For this review, use the dimensioned drawing (mm, ordinates from the lowest corner) and the shaded views. Give positions to 0.01 mm unless a question says otherwise; leave off trailing zeros. Loops run counter-clockwise (first coordinate to the right, second up) from the corner with the lowest first, then second, coordinate; pieces in that order, holes last. Notation, with made-up numbers: (66.25, -23.75) -> (90.25, -23.75) arc R19 ccw to (90.25, -5.75) -> close; hole circle Ø1 at (82, -29.5). An arc over 180 degrees is marked (long way). Use a Markdown table: item, result. Add a question column.
1. Add section B-B (y = 6.3). State the section outline as (x, z) points, and give its area (3 significant figures).
2. For pin 1 Ø4 at (y, z) = (8.5, 6.5) entering from -X; pin 2 Ø1.5 at (x, z) = (6, 2.5) entering from -Y; pin 3 Ø1.8 at (y, z) = (6.3, 7) entering from +X; pin 4 Ø1 at (y, z) = (6, 6) entering from -X, all flat-tipped, find the tip position at first contact; note any pin that passes through.
3. Add section D-D (y = 9). State the section outline as (x, z) points, and give its area (3 significant figures).
4. To check wall thickness, follow line 1 (Y direction, x = 6.75, z = 7); line 2 (Z direction, x = 3.75, y = 6.3); line 3 (X direction, y = 2, z = 5.5). State the ranges of each line that lie inside material, in increasing order.
5. Add section C-C (x = 6.75). State the section outline as (y, z) points.
6. Add section A-A (z = 7). State the section outline as (x, y) points, and give its area (3 significant figures).
7. Draft analysis for pull direction Y (two halves, no side actions). For the marked faces 1, 2 and 3, state which applies: pulls with the +Y half, pulls with the -Y half, needs draft (parallel to the pull), parting line crosses it, or undercut.
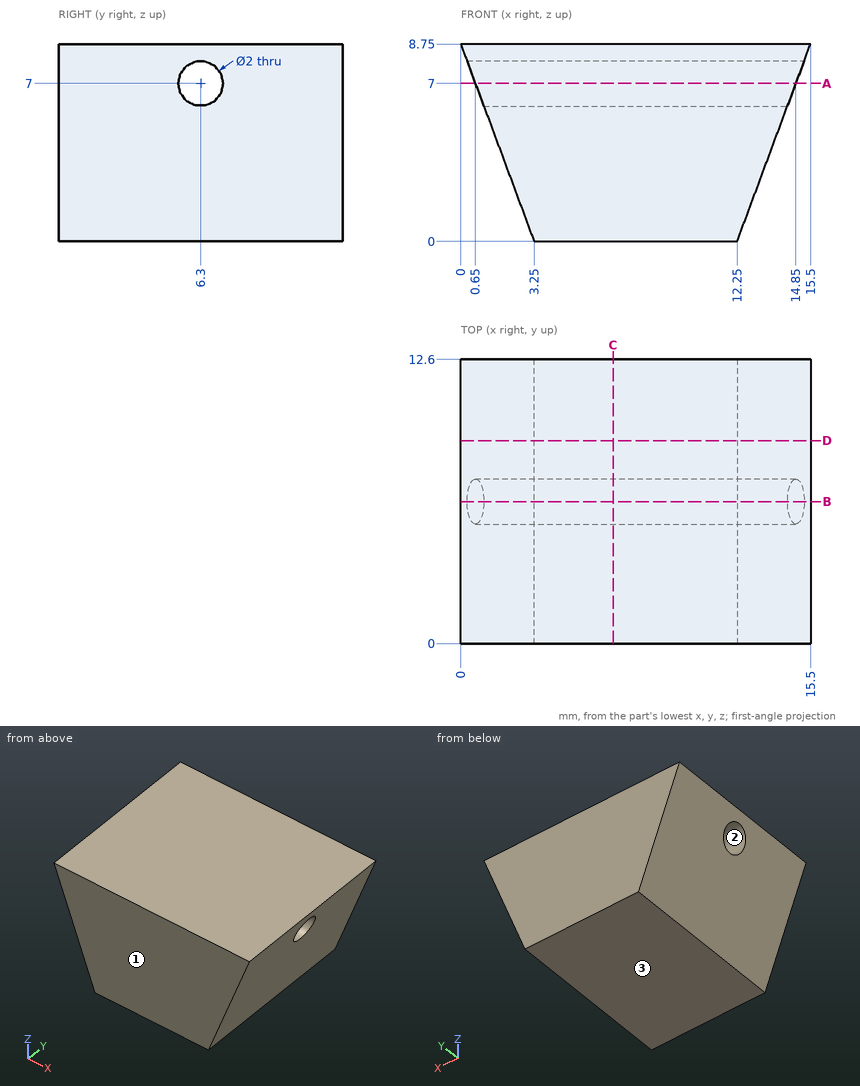
Taken from the geometry:
| question | item | result |
|---|---|---|
| 1 | outline | (0, 8.75) -> (0.28, 8) -> (15.22, 8) -> (15.5, 8.75) -> close; (1.02, 6) -> (3.25, 0) -> (12.25, 0) -> (14.48, 6) -> close |
| 1 | area | 78.8 mm^2 |
| 2 | pin 1 | stops at x = 0.09 |
| 2 | pin 2 | stops at y = 0 |
| 2 | pin 3 | passes through |
| 2 | pin 4 | stops at x = 0.91 |
| 3 | outline | (0, 8.75) -> (3.25, 0) -> (12.25, 0) -> (15.5, 8.75) -> close |
| 3 | area | 107 mm^2 |
| 4 | line 1 | y = 0 to 5.3, 7.3 to 12.6 |
| 4 | line 2 | z = 0 to 6, 8 to 8.75 |
| 4 | line 3 | x = 1.21 to 14.29 |
| 5 | outline | (0, 0) -> (12.6, 0) -> (12.6, 8.75) -> (0, 8.75) -> close; hole circle Ø2 at (6.3, 7) |
| 6 | outline | (0.65, 0) -> (14.85, 0) -> (14.85, 5.3) -> (0.65, 5.3) -> close; (0.65, 7.3) -> (14.85, 7.3) -> (14.85, 12.6) -> (0.65, 12.6) -> close |
| 6 | area | 151 mm^2 |
| 7 | face 1 | pulls with the -Y half |
| 7 | face 2 | undercut |
| 7 | face 3 | needs draft |
